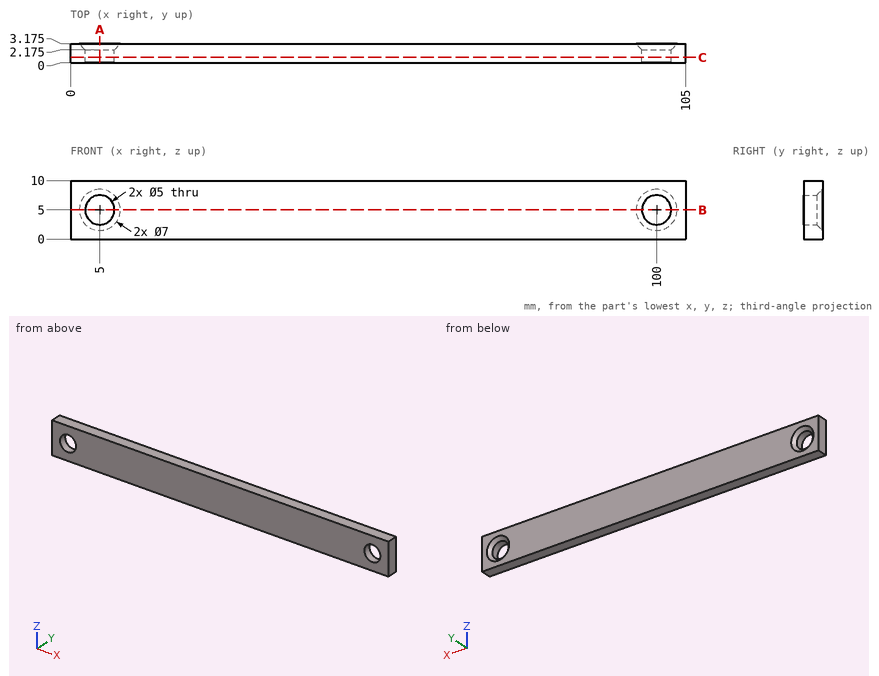
Design review of the part shown in the three views and the two pictorial views. Dimensions are in mm from the part's minimum x, y and z. Coordinates: 2 decimals unless noted, no trailing zeros. Loops run counter-clockwise (first coordinate to the right, second up) from the corner with the lowest first, then second, coordinate; pieces in that order, holes last. Notation, with made-up numbers: M 46.25,79 L 100.25,79 A14 cw 100.25,100 Z; hole C -10,61 d5. An arc over 180 degrees is marked long. Put each result on its own line as item: value. Start each with the question number.
Q1. Clearance check with flat-ended pins moving along their axes: pin 1 (4 mm diameter, centred on x = 5, z = 5, fed in from -Y); pin 2 (6 mm diameter, centred on x = 100, z = 5, fed in from +Y) (3 decimals). State where each tip first meets the part, or that it passes through.
Q2. Add section B-B (z = 5). Write out the cut boundary in (x, y) (3 decimals), and give its area (3 significant figures).
Q3. Add section A-A (x = 5). Write out the cut boundary in (y, z) (3 decimals), and give its area (3 significant figures).
Q4. Wall thickness on line 1 (X direction, y = 1.35, z = 5); line 2 (Z direction, x = 100, y = 0.9); line 3 (X direction, y = 0.25, z = 3.75): over which ranges is each line inside the solid? List them lowest first.
Q5. Add section C-C (y = 0.9). Write out the cut boundary in (x, z).
Answers:
1. pin 1: passes through
1. pin 2: stops at y = 2.675
2. outline: M 0,0 L 2.5,0 L 2.5,2.175 L 1.5,3.175 L 0,3.175 Z; M 7.5,0 L 97.5,0 L 97.5,2.175 L 96.5,3.175 L 8.5,3.175 L 7.5,2.175 Z; M 102.5,0 L 105,0 L 105,3.175 L 103.5,3.175 L 102.5,2.175 Z
2. area: 300 mm^2
3. outline: M 0,0 L 3.175,0 L 3.175,1.5 L 2.175,2.5 L 0,2.5 Z; M 0,7.5 L 2.175,7.5 L 3.175,8.5 L 3.175,10 L 0,10 Z
3. area: 14.9 mm^2
4. line 1: x = 0 to 2.5, 7.5 to 97.5, 102.5 to 105
4. line 2: z = 0 to 2.5, 7.5 to 10
4. line 3: x = 0 to 2.83, 7.17 to 97.83, 102.17 to 105
5. outline: M 0,0 L 105,0 L 105,10 L 0,10 Z; hole C 5,5 d5; hole C 100,5 d5
